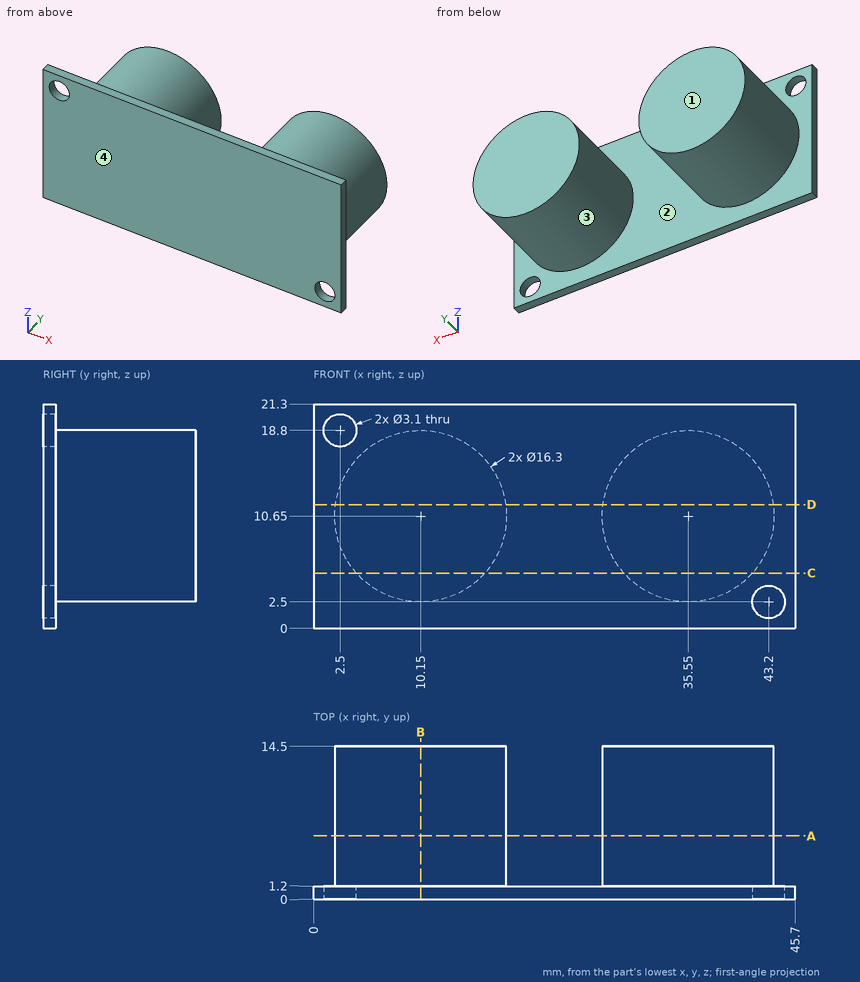
Verification items for this drawing (mm, ordinates from the low corner). A direction names the side the tool comes from. Round coordinates to 2 decimals unless told otherwise and drop trailing zeros. Write each loop counter-clockwise with the first axis right and the second up, starting at its lowest first coordinate (ties: lowest second). Pieces come first, ordered by that corner, then holes. Notation, with made-up numbers: (52.5, -27.75) - (105.5, -27.75) arc R31 cw to (105.5, 10.25) - close; hole circle Ø5 at (83.5, 33). An arc over 180 degrees is marked (long way). One line per item, written item: value.
1. Set-up check for the marked faces 1 and 2: record each of +Z, -Z, +X, -X, +Y, -Y from which the full face is reachable in a straight line by a thin tool's end or side.
The answers:
face 1: +Z, -Z, +X, -X, +Y
face 2: +Y
2. Scan lines: L1, parallel to X at y = 0.65, z = 2.5; L2, parallel to X at y = 0.4, z = 18.8; L3, parallel to Z at x = 43.2, y = 0.45. Record each from-to range of solid material in increasing order.
The answers:
L1: x = 0 to 41.65, 44.75 to 45.7
L2: x = 0 to 0.95, 4.05 to 45.7
L3: z = 0 to 0.95, 4.05 to 21.3
3. Cross-section at D-D on z = 11.75. Record the boundary of the cut face in (x, y), and give its area (3 significant figures).
The answers:
outline: (0, 0) - (45.7, 0) - (45.7, 1.2) - (43.63, 1.2) - (43.63, 14.5) - (27.47, 14.5) - (27.47, 1.2) - (18.23, 1.2) - (18.23, 14.5) - (2.07, 14.5) - (2.07, 1.2) - (0, 1.2) - close
area: 484 mm^2
4. Cross-section at A-A on y = 6. Record the boundary of the cut face in (x, z).
The answers:
outline: circle Ø16.3 at (10.15, 10.65); circle Ø16.3 at (35.55, 10.65)
5. Mould release check, pull along X, two halves, no side actions. Record for the marked faces 3 and 4: released by +X, released by -X, zero draft, split by the parting line, or undercut.
The answers:
face 3: undercut
face 4: zero draft
6. Depth check by flat-ended pin: pin 1 Ø1 at (x, z) = (22, 9.5) entering from -Y; pin 2 Ø1.5 at (x, y) = (13, 3.5) entering from +Z; pin 3 Ø4 at (y, z) = (6.5, 13) entering from +X; pin 4 Ø2.5 at (x, z) = (2.5, 18.8) entering from +Y. Enter the tip coordinate at first touch or a pass-through.
The answers:
pin 1: stops at y = 0
pin 2: stops at z = 18.52
pin 3: stops at x = 43.69
pin 4: passes through
7. Cross-section at C-C on z = 5.25. Record the boundary of the cut face in (x, y).
The answers:
outline: (0, 0) - (45.7, 0) - (45.7, 1.2) - (41.65, 1.2) - (41.65, 14.5) - (29.45, 14.5) - (29.45, 1.2) - (16.25, 1.2) - (16.25, 14.5) - (4.05, 14.5) - (4.05, 1.2) - (0, 1.2) - close
8. Cross-section at B-B on x = 10.15. Record the boundary of the cut face in (y, z), and give its area (3 significant figures).
The answers:
outline: (0, 0) - (1.2, 0) - (1.2, 2.5) - (14.5, 2.5) - (14.5, 18.8) - (1.2, 18.8) - (1.2, 21.3) - (0, 21.3) - close
area: 242 mm^2
